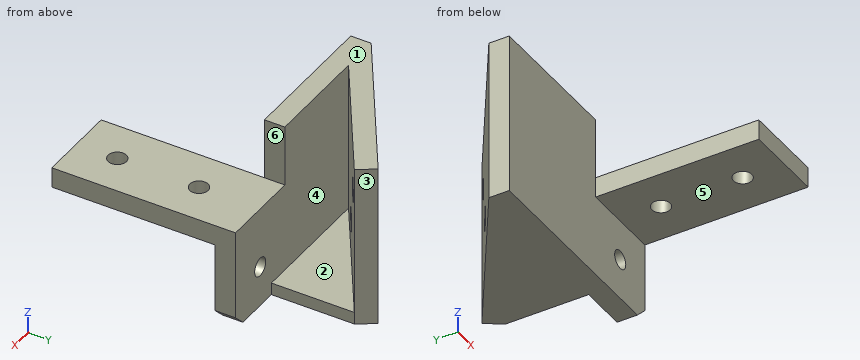
from build123d import *

# Parameters (mm, degrees)
SKETCH1_W           = 20
SKETCH1_H           = 20
SKETCH1_R           = 2.25
BOSS_EXTRUDE1_DEPTH = 5
SKETCH2_W           = 20
SKETCH2_H           = 45
SKETCH2_R           = 2.25
BOSS_EXTRUDE2_DEPTH = 5
CHAMFER1_SIZE       = 3
SKETCH3_W           = 40
SKETCH3_H           = 5
BOSS_EXTRUDE3_DEPTH = 35
BOSS_EXTRUDE4_DEPTH = 40
BOSS_EXTRUDE5_DEPTH = 3
CUT_EXTRUDE1_REACH  = 72.766
SKETCH6_R           = 2.75


with BuildPart() as part:
    # Sketch1 → Boss-Extrude1 (new body)
    with BuildSketch(Plane(origin=(0, 0, 0), x_dir=(1, 0, 0), z_dir=(0, 1, 0))):
        with Locations((10, 10)):
            Rectangle(SKETCH1_W, SKETCH1_H)
        with Locations(Location((10, 10, 0), (0, 0, 270))):
            Circle(SKETCH1_R, mode=Mode.SUBTRACT)
    extrude(amount=BOSS_EXTRUDE1_DEPTH)

    # Sketch2 → Boss-Extrude2 (add)
    with BuildSketch(Plane.XY):
        with Locations((10, -17.5)):
            Rectangle(SKETCH2_W, SKETCH2_H)
        with Locations((10, -30)):
            Circle(SKETCH2_R, mode=Mode.SUBTRACT)
        with Locations((10, -10)):
            Circle(SKETCH2_R, mode=Mode.SUBTRACT)
    extrude(amount=BOSS_EXTRUDE2_DEPTH)

    # Chamfer1
    chamfer1_edges = [part.edges().sort_by_distance(p)[0] for p in [
        (20, 2.5, -20),
    ]]
    chamfer(chamfer1_edges, length=CHAMFER1_SIZE)

    # Sketch3 → Boss-Extrude3 (add)
    with BuildSketch(Plane.ZY):
        with Locations((0, 2.5)):
            Rectangle(SKETCH3_W, SKETCH3_H)
    extrude(amount=BOSS_EXTRUDE3_DEPTH)

    # Sketch4 → Boss-Extrude4 (add)
    with BuildSketch(Plane.XY.offset(20)):
        Polygon((-35, 5), (2.740175558, 29.508756576), (5.463370733, 25.315403736), (-25.819607706, 5), align=None)
    extrude(amount=-BOSS_EXTRUDE4_DEPTH)

    # Sketch5 → Boss-Extrude5 (add)
    with BuildSketch(Plane(origin=(0, 0, -20), x_dir=(-1, 0, 0), z_dir=(0, 0, -1))):
        Polygon((-5.463370733, 25.315403736), (-5.463370733, 5), (25.819607706, 5), align=None)
    extrude(amount=-BOSS_EXTRUDE5_DEPTH)

    # Sketch6 → Cut-Extrude1 (cut, up to next)
    with BuildSketch(Plane(origin=(-12.66597239, 19.503887116, 0), x_dir=(0.8386705679454272, 0.5446390350150224, 0), z_dir=(-0.5446390350150224, 0.8386705679454272, 0)), mode=Mode.PRIVATE) as cut_extrude1_sk1:
        with Locations(Location((9.369725297, -8.25, 0), (0, 0, 180))):
            Circle(SKETCH6_R)
    cut_extrude1_tool1 = extrude(cut_extrude1_sk1.sketch, amount=-CUT_EXTRUDE1_REACH, mode=Mode.PRIVATE) & part.part
    # Sketch6 → Cut-Extrude1 (cut, up to next)
    with BuildSketch(Plane(origin=(-12.66597239, 19.503887116, 0), x_dir=(0.8386705679454272, 0.5446390350150224, 0), z_dir=(-0.5446390350150224, 0.8386705679454272, 0)), mode=Mode.PRIVATE) as cut_extrude1_sk2:
        with Locations(Location((-2.480274703, 8, 0), (0, 0, 180))):
            Circle(SKETCH6_R)
    cut_extrude1_tool2 = extrude(cut_extrude1_sk2.sketch, amount=-CUT_EXTRUDE1_REACH, mode=Mode.PRIVATE) & part.part
    add(cut_extrude1_tool1.solids().sort_by_distance((-4.80786, 24.607005, 8.25))[0], mode=Mode.SUBTRACT)
    add(cut_extrude1_tool2.solids().sort_by_distance((-14.746106, 18.153033, -8))[0], mode=Mode.SUBTRACT)


solid = part.part
Input: part model. Units: mm. Frame: model coordinates. Face numbers are marked on the shaded views. A direction names the side the tool comes from. Give positions to 0.01 mm unless a question says otherwise; leave off trailing zeros. Write each loop counter-clockwise with the first axis right and the second up, starting at its lowest first coordinate (ties: lowest second). Pieces come first, ordered by that corner, then holes.
Q1. Pull-direction query (Y, two-part tool) for the marked faces 1, 2 and 3; classes: pulls with the +Y half, pulls with the -Y half, needs draft (parallel to the pull), parting line crosses it, or undercut.
Q2. Section B-B, the plane y = -30. Output: boundary loops of the cut face in (x, z).
Q3. Set-up query: the marked faces 4, 5 and 6. Return all of +Z, -Z, +X, -X, +Y, -Y with unobstructed straight access to the full face (end or side cutting, diameter ignored); none if empty.
Q4. First-contact query: P1, Ø5, axis at x = -1.5, z = -11, coming from the +Y side; P2, Ø6, axis at x = 10, z = -10, coming from the -Y side; P3, Ø6, axis at y = -14, z = -0.5, coming from the -X side; P4, Ø22.5, axis at x = -5, y = 16, coming from the +Z side. Flat tips, straight axial feed; report the tip coordinate or a pass-through.
Q5. Material intervals for probe 1 along Y at (x, z) = (10, 1.9); probe 2 along X at (y, z) = (2, 13); probe 3 along Y at (x, z) = (15, -5), sorted ascending.
Q6. Section D-D, the plane z = 6.5. Output: boundary loops of the cut face in (x, y).
Q7. Section C-C, the plane z = -3.5. Output: boundary loops of the cut face in (x, y).
Q8. Section A-A, the plane x = 10. Output: boundary loops of the cut face in (y, z).
Filled in:
1. face 1: needs draft
1. face 2: undercut
1. face 3: pulls with the +Y half
2. outline: (0, 0) - (7.75, 0) - (7.75, 5) - (0, 5) - close; (12.25, 0) - (20, 0) - (20, 5) - (12.25, 5) - close
3. face 4: +Z, +X
3. face 5: -Z, +X, -X, -Y
3. face 6: +Z, +X, -Y
4. P1: stops at y = 28.38
4. P2: stops at y = 0
4. P3: stops at x = 0
4. P4: stops at z = 20
5. probe 1: y = -40 to -32.25, -27.75 to -12.25, -7.75 to 5
5. probe 2: x = -35 to 0
5. probe 3: y = 0 to 5
6. outline: (-35, 0) - (0, 0) - (0, 5) - (-25.82, 5) - (-3.86, 19.26) - (-6.59, 23.45) - (-35, 5) - close; (-3.03, 25.76) - (-0.31, 21.57) - (5.46, 25.32) - (2.74, 29.51) - close
7. outline: (-35, 0) - (20, 0) - (20, 5) - (-25.82, 5) - (5.46, 25.32) - (2.74, 29.51) - (-35, 5) - close
8. outline: (-40, 0) - (-32.25, 0) - (-32.25, 5) - (-40, 5) - close; (-27.75, 0) - (-12.25, 0) - (-12.25, 5) - (-27.75, 5) - close; (-7.75, 0) - (0, 0) - (0, -7.75) - (5, -7.75) - (5, 5) - (-7.75, 5) - close; (0, -20) - (5, -20) - (5, -12.25) - (0, -12.25) - close
